Here's how the part is built. I have some questions about the finished solid (model axes, mm). A direction names the side the tool comes from. Give positions to 0.01 mm unless a question says otherwise; leave off trailing zeros. Write each loop counter-clockwise with the first axis right and the second up, starting at its lowest first coordinate (ties: lowest second). Pieces come first, ordered by that corner, then holes. Notation, with made-up numbers: (13.25, 7) - (42.25, 7) arc R15 cw to (42.25, 36) - close; hole circle Ø6 at (78, 59). An arc over 180 degrees is marked (long way). Use a Markdown table: item, result.
Autodesk Fusion 360 part; units mm, degrees
sketch "Sketch1" plane through (0, 0, 0) normal (0, 0, 1) x (1, 0, 0)
  line L0 (0, 0) -> (60, 0)
  line L1 (0, 0) -> (0, -85)
  line L2 (0, -85) -> (60, -85)
  line L3 (60, -85) -> (60, 0)
  line L4 (30, -10) -> (46.75, -10)
  line L5 (46.75, -10) -> (13.25, -10)
  line L6 (13.25, -10) -> (13.25, -43.5)
  line L7 (13.25, -43.5) -> (46.75, -43.5)
  line L8 (46.75, -43.5) -> (46.75, -10)
  circle A0 centre (30, -65) radius 13
  line L9 (62, -87) -> (-2, -87)
  line L10 (-2, -87) -> (-2, 2)
  line L11 (-2, 2) -> (62, 2)
  line L12 (62, 2) -> (62, -87)
  dimension "d1" = 60
  dimension "d2" = 85
  dimension "d3" = 60
  dimension "d4" = 16.75
  dimension "d5" = 33.5
  dimension "d6" = 33.5
  dimension "d7" = 33.5
  dimension "d8" = 26
extrude "Extrude1" add sketch "Sketch1" against normal blind 3 contours L0 L1 L2 L3 | L9 L10 L11 L12
extrude "Extrude2" add sketch "Sketch1" against normal blind 12 contours L9 L10 L11 L12
fillet "Fillet1" radius 2 4 edges at (-2, -42.5, 0) (30, 2, 0) (62, -42.5, 0) (30, -87, 0)
Item 1: I need wall thicknesses on line 1 along Y through (x, z) = (30, -2.4); line 2 along X through (y, z) = (-58.5, -8); line 3 along Y through (x, z) = (30, -1.4). Which ranges of each line are inside material? Lowest first, please. Write a range as [from, to].
Values:
| item | result |
|---|---|
| line 1 | y = [-87, -78], [-52, -43.5], [-10, 2] |
| line 2 | x = [-2, 0], [60, 62] |
| line 3 | y = [-86.91, -78], [-52, -43.5], [-10, 1.91] |
Item 2: For faces 1 (the flat face through (30, -10, -1)), 2 (the flat face through (62, -42, -7)), 3 (the flat face through (30, 0, -7)), which set-ups out of +Z, -Z, +X, -X, +Y, -Y let a thin tool reach every point of the face, with its end or its side?
Values:
| item | result |
|---|---|
| face 1 | +Z, -Z |
| face 2 | +Z, -Z, +X, +Y, -Y |
| face 3 | -Z |
Item 3: If we section it at A-A, the plane x = 45: Write out the boundary of the cut face in (y, z).
Values:
| item | result |
|---|---|
| outline | (-87, -12) - (-85, -12) - (-85, -3) - (-43.5, -3) - (-43.5, 0) - (-85, 0) arc R2 ccw to (-87, -2) - close; (-10, -3) - (0, -3) - (0, -12) - (2, -12) - (2, -2) arc R2 ccw to (0, 0) - (-10, 0) - close |
Item 4: Thinking about a two-plate mould opening in Y: for faces 4 (the cylindrical face through (-1.43, -41.88, -0.6)), 5 (the flat face through (30, -51, -3)), 6 (the cylindrical face through (29.55, -86.43, -0.6)), 7 (the flat face through (60, -43, -7)), which applies, +Y half, -Y half, draft (parallel to the pull), parting line (faces both ways), or undercut?
Values:
| item | result |
|---|---|
| face 4 | draft |
| face 5 | undercut |
| face 6 | -Y half |
| face 7 | undercut |
Item 5: If we section it at D-D, the plane x = 23: Write out the boundary of the cut face in (y, z).
Values:
| item | result |
|---|---|
| outline | (-87, -12) - (-85, -12) - (-85, -3) - (-75.95, -3) - (-75.95, 0) - (-85, 0) arc R2 ccw to (-87, -2) - close; (-54.05, -3) - (-43.5, -3) - (-43.5, 0) - (-54.05, 0) - close; (-10, -3) - (0, -3) - (0, -12) - (2, -12) - (2, -2) arc R2 ccw to (0, 0) - (-10, 0) - close |
Item 6: If we section it at B-B, the plane z = -6.25: Write out the boundary of the cut face in (x, y).
Values:
| item | result |
|---|---|
| outline | (-2, -87) - (62, -87) - (62, 2) - (-2, 2) - close; hole (0, -85) - (60, -85) - (60, 0) - (0, 0) - close |
Item 7: If we section it at C-C, the plane y = -65: Write out the boundary of the cut face in (x, z).
Values:
| item | result |
|---|---|
| outline | (-2, -12) - (0, -12) - (0, -3) - (17, -3) - (17, 0) - (0, 0) arc R2 ccw to (-2, -2) - close; (43, -3) - (60, -3) - (60, -12) - (62, -12) - (62, -2) arc R2 ccw to (60, 0) - (43, 0) - close |
